Geometry check sheet. Reference: the model listing, model coordinates, mm. A direction names the side the tool comes from. Round coordinates to 2 decimals unless told otherwise and drop trailing zeros. Write each loop counter-clockwise with the first axis right and the second up, starting at its lowest first coordinate (ties: lowest second). Pieces come first, ordered by that corner, then holes. Notation, with made-up numbers: (64, 63) -> (68, 63) arc R24 ccw to (68, 102) -> close; hole circle Ø3 at (30.5, 77). An arc over 180 degrees is marked (long way). Return JSON: item names as keys, results as strings. Group by question number.
Solid Edge part; units mm, degrees
sketch "Sketch1" plane through (0, 0, 0) normal (0, 0, 1) x (1, 0, 0)
  arc A0 (-81.6347, -15) -> (-80.3868, 14.948) centre (-81.6347, 0) cw
  line L0 (-80.3868, 14.948) -> (38.3653, 10)
  arc A1 (38.3653, 10) -> (38.3653, -10) centre (38.3653, 0) cw
  line L1 (38.3653, -10) -> (-81.6347, -15)
  circle A2 centre (38.3653, 0) radius 5
  circle A3 centre (-81.6347, 0) radius 10
extrude "Protrusion1" add sketch "Sketch1" along normal blind 15
sketch "Sketch2" plane through (-24.1347, 0, 31.5) normal (0, 0, 1) x (0.9991331, 0.0416305, 0)
  circle A0 centre (62.4537, -2.6022) radius 5.0079
extrude "ExtrudedProtrusion_3" add sketch "Sketch2" against normal blind 48
1) Material ranges on probe 1 along Z at (x, y) = (-58, -10.5); probe 2 along X at (y, z) = (-8, 12); probe 3 along Y at (x, z) = (-89.5, 9.5), recorded low to high. Write a range as [from, to].
2) Go/stop test with flat-tipped pins: P1, Ø5, axis at x = -58, z = 9.5, coming from the +Y side; P2, Ø1, axis at x = -22, y = 1.5, coming from the -Z side; P3, Ø2, axis at x = -48.5, z = 7, coming from the -Y side. Record where each tip stops, or that it passes through.
3) Sectioned sample at A-A on z = 12. Enter the section's corners in (x, y).
4) Tool access check on faces 4 (the face through (-21.84, 12.51, 7.4)), 5 (the face through (33.365, 0.012, 23.366)), 6 (the face through (33.365, 0.012, -8.135)). Record the directions out of +Z, -Z, +X, -X, +Y, -Y that give a thin tool (end or side, any length) a straight path to the whole face; none if there is none.
5) Sectioned sample at B-B on y = 3.5. Enter the section's corners in (x, z) (3 decimals), and give its area (3 significant figures).
6) Mould release check, pull along Y, two halves, no side actions. Record for faces 1 (the face through (-23, 0, 0)), 2 (the face through (-72.096, -3.004, 7.395)), 3 (the face through (-96.63, 0.29, 7.4)): +Y half, -Y half, draft (parallel to the pull), parting line (faces both ways), or undercut.
7) Sectioned sample at C-C on x = -88. Enter the section's corners in (y, z).
8) Sectioned sample at D-D on y = -13. Enter the section's corners in (x, z).
Evaluation:
{
 "1": {"probe 1": "z = [0, 15]", "probe 2": "x = [-94.32, -87.63], [-75.63, 44.37]", "probe 3": "y = [-12.77, -6.18], [6.18, 12.77]"},
 "2": {"P1": "stops at y = 14.12", "P2": "stops at z = 0", "P3": "stops at y = -13.66"},
 "3": {"outline": "(-81.63, -15) -> (38.37, -10) arc R10 ccw to (38.37, 10) -> (-80.39, 14.95) arc R15 ccw (long way) to start; hole circle Ø20 at (-81.63, 0)"},
 "4": {"face 4": "+Z, -Z, +X, +Y", "face 5": "+Z", "face 6": "-Z"},
 "5": {"outline": "(-96.221, 0) -> (-91.002, 0) -> (-91.002, 15) -> (-96.221, 15) -> close; (-72.267, 0) -> (34.791, 0) -> (34.791, -16.5) -> (41.955, -16.5) -> (41.955, 0) -> (47.733, 0) -> (47.733, 15) -> (41.955, 15) -> (41.955, 31.5) -> (34.791, 31.5) -> (34.791, 15) -> (-72.267, 15) -> close", "area": "2,110 mm2"},
 "6": {"face 1": "draft", "face 2": "undercut", "face 3": "parting line"},
 "7": {"outline": "(-13.58, 0) -> (-7.71, 0) -> (-7.71, 15) -> (-13.58, 15) -> close; (7.71, 0) -> (13.58, 0) -> (13.58, 15) -> (7.71, 15) -> close"},
 "8": {"outline": "(-89.12, 0) -> (-33.63, 0) -> (-33.63, 15) -> (-89.12, 15) -> close"}
}
